from build123d import *

# Parameters (mm, degrees)
SKETCH1_W           = 120
SKETCH1_H           = 20
BOSS_EXTRUDE1_DEPTH = 8
SKETCH2_W           = 8
SKETCH2_H           = 20
BOSS_EXTRUDE2_DEPTH = 10
SKETCH3_R           = 1.75
CUT_EXTRUDE1_DEPTH  = 10


with BuildPart() as part:
    # Sketch1 → Boss-Extrude1 (new body)
    with BuildSketch(Plane(origin=(0, 0, 0), x_dir=(1, 0, 0), z_dir=(0, 1, 0))):
        Rectangle(SKETCH1_W, SKETCH1_H)
    extrude(amount=BOSS_EXTRUDE1_DEPTH)

    # Sketch2 → Boss-Extrude2 (add)
    with BuildSketch(Plane.XZ):
        with Locations((56, 0)):
            Rectangle(SKETCH2_W, SKETCH2_H)
        with Locations((-56, 0)):
            Rectangle(SKETCH2_W, SKETCH2_H)
    extrude(amount=BOSS_EXTRUDE2_DEPTH)

    # Sketch3 → Cut-Extrude1 (cut)
    with BuildSketch(Plane.XZ):
        with Locations((32.5, 0)):
            Circle(SKETCH3_R)
        with Locations((-32.5, 0)):
            Circle(SKETCH3_R)
    extrude(amount=-CUT_EXTRUDE1_DEPTH, mode=Mode.SUBTRACT)


solid = part.part
Read the model definition and answer for the solid it produces. Units are mm, in the model's axes. A direction names the side the tool comes from. Give positions to 0.01 mm unless a question says otherwise; leave off trailing zeros. Write each loop counter-clockwise with the first axis right and the second up, starting at its lowest first coordinate (ties: lowest second). Pieces come first, ordered by that corner, then holes. Notation, with made-up numbers: (7, 43.25) - (64, 43.25) arc R12 cw to (64, 66.25) - close; hole circle Ø1 at (82.5, 51.5). An arc over 180 degrees is marked (long way). Use CSV: the item, a comma, the result in double quotes. Start each with the question number.
(1) Find section B-B (y = -8.5). Give the vertices of the cut face in (x, z), plus the area to 3 significant figures.
(2) Given P1, Ø3, axis at x = 32.5, z = 0, coming from the +Y side; P2, Ø4.5, axis at x = -32.5, z = 0, coming from the +Y side, each flat-ended and moving along its own axis, determine where each tip first touches the part or whether it passes through.
(3) Find section A-A (z = 0). Give the vertices of the cut face in (x, y).
(4) Find section D-D (z = 9). Give the vertices of the cut face in (x, y).
(5) Consider line 1 along X through (y, z) = (-7, -3.5); line 2 along Z through (x, y) = (32.5, 3.5); line 3 along X through (y, z) = (0.5, 1.5). Determine where each line is inside the solid, lowest interval first.
(6) For faces 4 (the flat face through (-1, 0, 0)), 5 (the flat face through (60, -1, 0)), determine the directions among +Z, -Z, +X, -X, +Y, -Y from which every point of the face is accessible in a straight line to the end or side of a thin tool.
(7) Find section C-C (x = -32.5). Give the vertices of the cut face in (y, z).
(8) Determine the mould class of faces 1 (the flat face through (-1, 3, 10)), 2 (the cylindrical face through (-34.25, 3.94, 0.08)), 3 (the flat face through (-52, -5, 0)) for opening direction Z: +Z half, -Z half, draft (parallel to the pull), parting line (faces both ways), or undercut.
Findings below:
1,outline,"(-60, -10) - (-52, -10) - (-52, 10) - (-60, 10) - close; (52, -10) - (60, -10) - (60, 10) - (52, 10) - close"
1,area,"320 mm2"
2,P1,"through"
2,P2,"y = 8"
3,outline,"(-60, -10) - (-52, -10) - (-52, 0) - (-34.25, 0) - (-34.25, 8) - (-60, 8) - close; (-30.75, 0) - (30.75, 0) - (30.75, 8) - (-30.75, 8) - close; (34.25, 0) - (52, 0) - (52, -10) - (60, -10) - (60, 8) - (34.25, 8) - close"
4,outline,"(-60, -10) - (-52, -10) - (-52, 0) - (52, 0) - (52, -10) - (60, -10) - (60, 8) - (-60, 8) - close"
5,line 1,"-60 to -52, 52 to 60"
5,line 2,"-10 to -1.75, 1.75 to 10"
5,line 3,"-60 to -33.4, -31.6 to 31.6, 33.4 to 60"
6,face 4,"+Z, -Z, -Y"
6,face 5,"+Z, -Z, +X, +Y, -Y"
7,outline,"(0, -10) - (8, -10) - (8, -1.75) - (0, -1.75) - close; (0, 1.75) - (8, 1.75) - (8, 10) - (0, 10) - close"
8,face 1,"+Z half"
8,face 2,"undercut"
8,face 3,"draft"
